The model under review builds one solid part; all positions refer to its coordinate system, in mm. Round coordinates to 2 decimals unless told otherwise and drop trailing zeros. Order: outer loops, then holes, each group sorted by start corner. A loop starts at its lowest first (then second) coordinate and runs counter-clockwise, first axis right, second up. Notation, with made-up numbers: M 78,-13.75 L 122,-13.75 A11 cw 122,3.25 Z; hole C 41.25,42 d5. An arc over 180 degrees is marked long. Use a Markdown table: item, result. Add a question column.
1. Consider section D-D on x = -97.5. State the section outline as (y, z) points.
2. Consider section A-A on y = 16.5. State the section outline as (x, z) points.
3. Insertion check: P1, Ø3, axis at x = -7.5, z = 3.5, coming from the +Y side; P2, Ø1.8, axis at x = -95, z = 2.5, coming from the -Y side; P3, Ø1.8, axis at x = -9, z = 2, coming from the -Y side; P4, Ø24, axis at x = -53.03, y = 7.7, coming from the +Z side. Each pin has a flat end and moves straight along its axis. Give the tip position at first contact, or say it passes through.
4. Consider section C-C on x = -69.5. State the section outline as (y, z) points.
5. To check wall thickness, follow probe 1 along Y at (x, z) = (-63, 5.55); probe 2 along X at (y, z) = (-7.5, 1.05); probe 3 along X at (y, z) = (26, 4). State the ranges of each line that lie inside material, in increasing order.
6. Consider section B-B on z = 2.3. State the section outline as (x, y) points.
from build123d import *

# Parameters (mm, degrees)
SKETCH1_R           = 20
BOSS_EXTRUDE1_DEPTH = 6


with BuildPart() as part:
    # Sketch1 → Boss-Extrude1 (new body)
    with BuildSketch(Plane.XY.offset(6)):
        with BuildLine():
            Line((-91.761844853, 17.703382647), (-101.518898091, 17.703382647))
            ThreePointArc((-101.518898091, 17.703382647), (-111.518898091, 7.703382647), (-101.518898091, -2.296617353))
            Line((-101.518898091, -2.296617353), (-91.761844853, -2.296617353))
            ThreePointArc((-91.761844853, -2.296617353), (-55.664437873, -32.209902495), (-15.951018956, -7.296617353))
            Line((-15.951018956, -7.296617353), (-1.518898091, -7.296617353))
            ThreePointArc((-1.518898091, -7.296617353), (5.552169721, -4.367685165), (8.481101909, 2.703382647))
            Line((8.481101909, 2.703382647), (8.481101909, 12.703382647))
            ThreePointArc((8.481101909, 12.703382647), (5.552169721, 19.774450459), (-1.518898091, 22.703382647))
            Line((-1.518898091, 22.703382647), (-15.951018956, 22.703382647))
            ThreePointArc((-15.951018956, 22.703382647), (-55.664437873, 47.616667789), (-91.761844853, 17.703382647))
        make_face()
        with Locations(Location((-53.032011391, 7.703382647, 0), (0, 0, 180))):
            Circle(SKETCH1_R, mode=Mode.SUBTRACT)
        with BuildLine():
            Line((-7.032011391, 10.953382647), (0.967988609, 10.953382647))
            ThreePointArc((0.967988609, 10.953382647), (4.217988609, 7.703382647), (0.967988609, 4.453382647))
            Line((0.967988609, 4.453382647), (-7.032011391, 4.453382647))
            ThreePointArc((-7.032011391, 4.453382647), (-10.282011391, 7.703382647), (-7.032011391, 10.953382647))
        make_face(mode=Mode.SUBTRACT)
    extrude(amount=-BOSS_EXTRUDE1_DEPTH)


solid = part.part
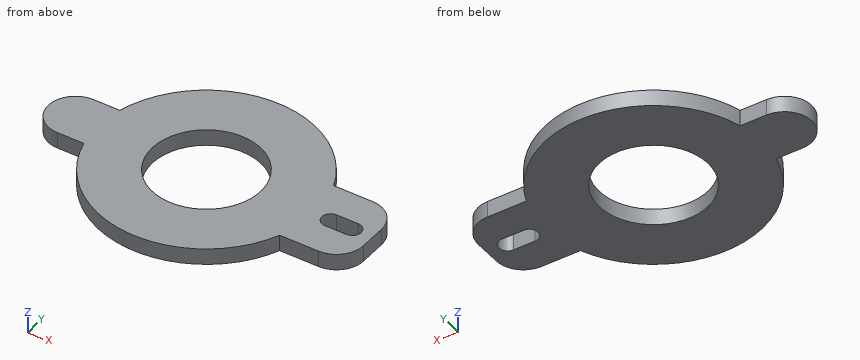
Answer block:
| question | item | result |
|---|---|---|
| 1 | outline | M -2.3,0 L 17.7,0 L 17.7,6 L -2.3,6 Z |
| 2 | outline | M -106.27,0 L -70.99,0 L -70.99,6 L -106.27,6 Z; M -35.07,0 L 7.73,0 L 7.73,6 L -35.07,6 Z |
| 3 | P1 | y = 22.7 |
| 3 | P2 | y = -2.3 |
| 3 | P3 | y = -7.3 |
| 3 | P4 | through |
| 4 | outline | M -28.75,0 L -3.65,0 L -3.65,6 L -28.75,6 Z; M 19.05,0 L 44.16,0 L 44.16,6 L 19.05,6 Z |
| 5 | probe 1 | -31.03 to -9.64, 25.04 to 46.44 |
| 5 | probe 2 | -90.03 to -66.03, -40.04 to -16.03 |
| 5 | probe 3 | -88.6 to -61.11, -44.96 to -17.46 |
| 6 | outline | M -101.52,-2.3 L -91.76,-2.3 A40 ccw -15.95,-7.3 L -1.52,-7.3 A10 ccw 8.48,2.7 L 8.48,12.7 A10 ccw -1.52,22.7 L -15.95,22.7 A40 ccw -91.76,17.7 L -101.52,17.7 A10 ccw Z; hole C -53.03,7.7 d40; hole M -7.03,4.45 L 0.97,4.45 A3.25 ccw 0.97,10.95 L -7.03,10.95 A3.25 ccw Z |
